from build123d import *


with BuildPart() as part:
    # Sketch1 → Revolve1 (revolve)
    with BuildSketch(Plane(origin=(0, 0, 0), x_dir=(1, 0, 0), z_dir=(0, 1, 0))):
        with BuildLine():
            Line((-19.177, 3), (19.177, 3))
            Line((19.177, 3), (19.177, 2))
            Line((19.177, 2), (19.917, 2))
            Line((19.917, 2), (19.917, 3))
            Line((19.917, 3), (20.8, 3))
            ThreePointArc((20.8, 3), (20.941421356, 2.941421356), (21, 2.8))
            Line((21, 2.8), (21, 0))
            Line((21, 0), (-21, 0))
            Line((-21, 0), (-21, 2.8))
            ThreePointArc((-21, 2.8), (-20.941421356, 2.941421356), (-20.8, 3))
            Line((-20.8, 3), (-19.917, 3))
            Line((-19.917, 3), (-19.917, 2))
            Line((-19.917, 2), (-19.177, 2))
            Line((-19.177, 2), (-19.177, 3))
        make_face()
    revolve(axis=Axis((21, 0, 0), (-1, 0, 0)))


solid = part.part
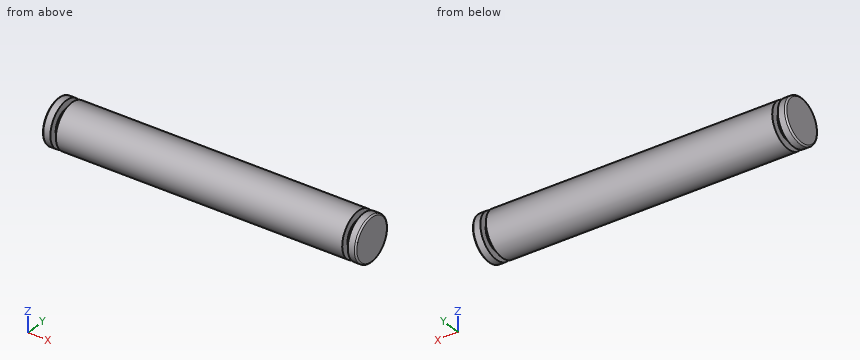
The model under review builds one solid part; all positions refer to its coordinate system, in mm. Round coordinates to 2 decimals unless told otherwise and drop trailing zeros. Loops run counter-clockwise (first coordinate to the right, second up) from the corner with the lowest first, then second, coordinate; pieces in that order, holes last. Notation, with made-up numbers: M -35.5,61.5 L -2.5,61.5 A29 ccw -2.5,95.5 Z; hole C 54.25,45.25 d8. An arc over 180 degrees is marked long. Answer as a JSON object with one key per item and string values.
Item 1: For line 1 along X through (y, z) = (-0.5, 2.25); line 2 along Y through (x, z) = (-1.5, 2.25); line 3 along Y through (x, z) = (5, -1.75), list the stretches that pass through material, from the lowest coordinate up.
Check sheet entries:
{"line 1": "-21 to -19.92, -19.18 to 19.18, 19.92 to 21", "line 2": "-1.98 to 1.98", "line 3": "-2.44 to 2.44"}
Item 2: Clearance check with flat-ended pins moving along their axes: P1, Ø2, axis at x = 8.5, z = 1.5, coming from the +Y side; P2, Ø1, axis at x = 14.5, y = -1, coming from the +Z side. State where each tip first meets the part, or that it passes through.
Check sheet entries:
{"P1": "y = 2.96", "P2": "z = 2.96"}
Item 3: We need section A-A, the plane x = -13.5. State the section outline as (y, z) points, and give its area (3 significant figures).
Check sheet entries:
{"outline": "C 0,0 d6", "area": "28.3 mm2"}
